Design review of the part shown in the three views and the two pictorial views. Dimensions are in mm from the part's minimum x, y and z. Give positions to 0.01 mm unless a question says otherwise; leave off trailing zeros. Loops run counter-clockwise (first coordinate to the right, second up) from the corner with the lowest first, then second, coordinate; pieces in that order, holes last.
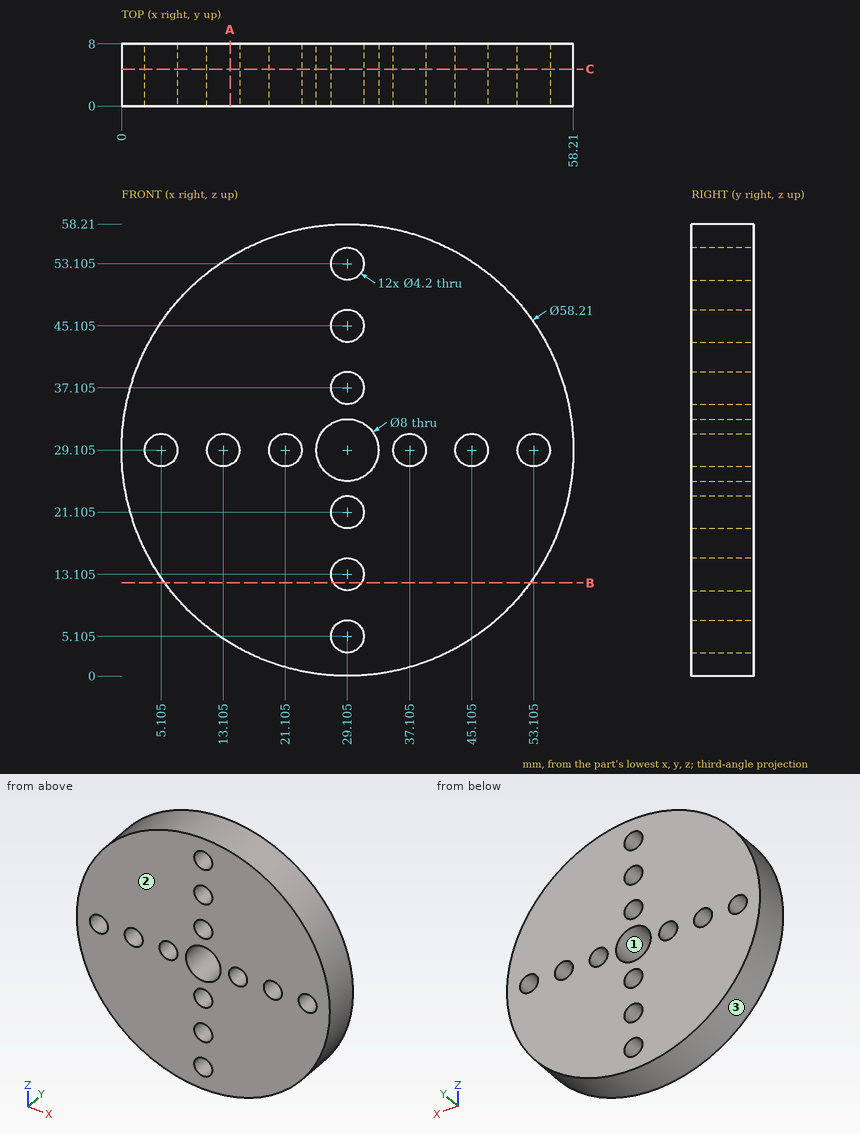
Q1. Take a section at C-C (y = 4.75). Give the number of separate pieces and of enclosed holes in the cut face, plus the area to 3 significant figures.
Results:
separate pieces: 1
enclosed holes: 13
area: 2,440 mm2
Q2. Take a section at B-B (z = 12). Give the boundary of the cut face in (x, y), plus the area to 3 significant figures.
Results:
outline: (5.56, 0) - (27.32, 0) - (27.32, 8) - (5.56, 8) - close; (30.89, 0) - (52.65, 0) - (52.65, 8) - (30.89, 8) - close
area: 348 mm2
Q3. Take a section at A-A (x = 14). Give the boundary of the cut face in (y, z).
Results:
outline: (0, 4.23) - (8, 4.23) - (8, 27.21) - (0, 27.21) - close; (0, 31) - (8, 31) - (8, 53.98) - (0, 53.98) - close
Q4. Draft analysis for pull direction X (two halves, no side actions). For the marked faces 1, 2 and 3, state which applies: pulls with the +X half, pulls with the -X half, needs draft (parallel to the pull), parting line crosses it, or undercut.
Results:
face 1: undercut
face 2: needs draft
face 3: parting line crosses it
Q5. Wall thickness on line 1 (X direction, y = 5.5, z = 26); line 2 (X direction, y = 6.25, z = 5); line 3 (Z direction, x = 13, y = 3.75): over which ranges is each line inside the solid? List them lowest first.
Results:
line 1: x = 0.17 to 26.58, 31.63 to 58.04
line 2: x = 12.79 to 27.01, 31.2 to 45.42
line 3: z = 4.86 to 27.01, 31.2 to 53.35
Q6. Insertion check: pin 1 (9 mm diameter, centred on x = 29.105, z = 29.105, fed in from -Y); pin 2 (3.5 mm diameter, centred on x = 29.105, z = 45.105, fed in from -Y); pin 3 (4 mm diameter, centred on x = 17, y = 1, fed in from -Z); pin 4 (1 mm diameter, centred on y = 4.5, z = 17, fed in from +X). Each pin has a flat end and moves straight along its axis. Give the tip position at first contact, or say it passes through.
Results:
pin 1: stops at y = 0
pin 2: passes through
pin 3: stops at z = 1.81
pin 4: stops at x = 55.8
